Input: part model. Units: mm. Frame: model coordinates. Face numbers are marked on the shaded views. A direction names the side the tool comes from. Round coordinates to 2 decimals unless told otherwise and drop trailing zeros. Write each loop counter-clockwise with the first axis right and the second up, starting at its lowest first coordinate (ties: lowest second). Pieces come first, ordered by that corner, then holes. Notation, with made-up numbers: M -31,77 L 21,77 A33 ccw 21,105 Z; hole C -22,86.25 d10. An arc over 180 degrees is marked long. Use one line per item in the form item = value. Start each with the question number.
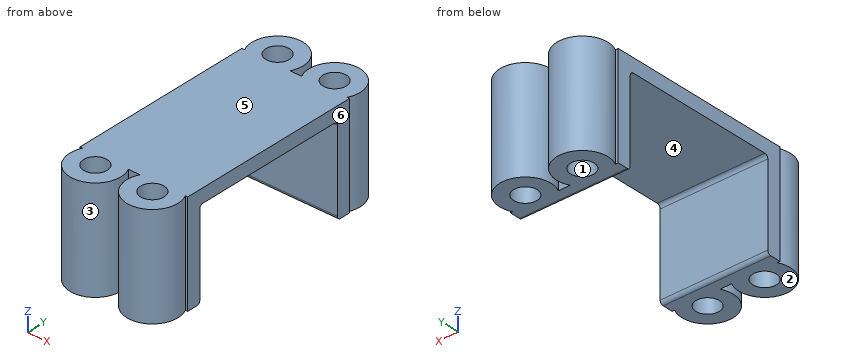
```python
from build123d import *

# Parameters (mm, degrees)
SCHIZZO1_W                   = 15.6
SCHIZZO1_H                   = 22.8
ESTRUSIONE_ESTRUSIONE1_DEPTH = 2
SCHIZZO7_R                   = 1.7
ESTRUSIONE_ESTRUSIONE8_DEPTH = 14.75
RACCORDO2_R                  = 0.5


with BuildPart() as part:
    # Schizzo1 → Estrusione-Estrusione1 (new body)
    with BuildSketch(Plane.XY):
        with Locations((-0.031567178, 0)):
            Rectangle(SCHIZZO1_W, SCHIZZO1_H)
    extrude(amount=ESTRUSIONE_ESTRUSIONE1_DEPTH)

    # Schizzo7 → Estrusione-Estrusione8 (add)
    # profile 1 of 2: a face of its own
    with BuildSketch(Plane.XY.offset(2)):
        with BuildLine():
            Line((7.768432822, 13.4), (7.417902523, 13.4))
            ThreePointArc((7.417902523, 13.4), (4.131567178, 18.8), (0.845231833, 13.4))
            Line((0.845231833, 13.4), (-0.845231833, 13.4))
            ThreePointArc((-0.845231833, 13.4), (-4.131567178, 18.8), (-7.417902523, 13.4))
            Line((-7.417902523, 13.4), (-7.831567178, 13.4))
            Line((-7.831567178, 13.4), (-7.831567178, 11.4))
            Line((-7.831567178, 11.4), (7.768432822, 11.4))
            Line((7.768432822, 11.4), (7.768432822, 13.4))
        make_face()
        with Locations((4.131567178, 15.1)):
            Circle(SCHIZZO7_R, mode=Mode.SUBTRACT)
        with Locations(Location((-4.131567178, 15.1, 0), (0, 0, 180))):
            Circle(SCHIZZO7_R, mode=Mode.SUBTRACT)
    # profile 2 of 2: a face of its own
    with BuildSketch(Plane.XY.offset(2)):
        with BuildLine():
            Line((0.845231833, -13.4), (-0.845231833, -13.4))
            ThreePointArc((-0.845231833, -13.4), (-4.131567178, -18.8), (-7.417902523, -13.4))
            Line((-7.417902523, -13.4), (-7.831567178, -13.4))
            Line((-7.831567178, -13.4), (-7.831567178, -11.4))
            Line((-7.831567178, -11.4), (7.768432822, -11.4))
            Line((7.768432822, -11.4), (7.768432822, -13.4))
            Line((7.768432822, -13.4), (7.417902523, -13.4))
            ThreePointArc((7.417902523, -13.4), (4.131567178, -18.8), (0.845231833, -13.4))
        make_face()
        with Locations((-4.131567178, -15.1)):
            Circle(SCHIZZO7_R, mode=Mode.SUBTRACT)
        with Locations(Location((4.131567178, -15.1, 0), (0, 0, 180))):
            Circle(SCHIZZO7_R, mode=Mode.SUBTRACT)
    extrude(amount=-ESTRUSIONE_ESTRUSIONE8_DEPTH)

    # Raccordo2
    raccordo2_edges = [part.edges().sort_by_distance(p)[0] for p in [
        (-0.031567178, 11.4, 0),
        (-0.031567178, 11.4, -12.75),
        (-0.031567178, -11.4, 0),
        (-0.031567178, -11.4, -12.75),
    ]]
    fillet(raccordo2_edges, radius=RACCORDO2_R)


solid = part.part
```
Item 1: Cut plane A-A (z = -1.75). Output: boundary loops of the cut face in (x, y), plus the area to 3 significant figures.
Item 2: Cut plane B-B (y = -15.1). Output: boundary loops of the cut face in (x, z).
Item 3: First-contact query: pin 1 (0.8 mm diameter, centred on x = 0, z = -5.5, fed in from -Y); pin 2 (8 mm diameter, centred on x = -4, y = 5, fed in from -Z); pin 3 (0.8 mm diameter, centred on x = 0, z = -5, fed in from +Y). Flat tips, straight axial feed; report the tip coordinate or a pass-through.
Item 4: Reachability of the marked faces 4, 5 and 6 from +Z, -Z, +X, -X, +Y, -Y: full face, straight path, thin tool, end or side. Return the list, or none.
Item 5: Cut plane C-C (x = -3.5). Output: boundary loops of the cut face in (y, z), plus the area to 3 significant figures.
Item 6: Ray query, line 1 (Y direction, x = 3.75, z = -1.25); line 2 (Z direction, x = 0.25, y = -9); line 3 (Y direction, x = -0.25, z = -10.25). Return the intervals inside material, ascending. Write a range as from..to.
Item 7: Draft query along Y for the marked faces 1, 2 and 3. Return one class per face: +Y half, -Y half, draft (parallel to the pull), parting line (faces both ways), or undercut.
Item 8: Cut plane D-D (x = 6.5). Output: boundary loops of the cut face in (y, z).
Final values:
q1.outline = M -7.83,-13.4 L -7.42,-13.4 A3.7 ccw long -0.85,-13.4 L 0.85,-13.4 A3.7 ccw long 7.42,-13.4 L 7.77,-13.4 L 7.77,-11.4 L -7.83,-11.4 Z; M -7.83,11.4 L 7.77,11.4 L 7.77,13.4 L 7.42,13.4 A3.7 ccw long 0.85,13.4 L -0.85,13.4 A3.7 ccw long -7.42,13.4 L -7.83,13.4 Z; hole C -4.13,-15.1 d3.4; hole C -4.13,15.1 d3.4; hole C 4.13,-15.1 d3.4; hole C 4.13,15.1 d3.4
q1.area = 161 mm^2
q2.outline = M -7.83,-12.75 L -5.83,-12.75 L -5.83,2 L -7.83,2 Z; M -2.43,-12.75 L -0.43,-12.75 L -0.43,2 L -2.43,2 Z; M 0.43,-12.75 L 2.43,-12.75 L 2.43,2 L 0.43,2 Z; M 5.83,-12.75 L 7.83,-12.75 L 7.83,2 L 5.83,2 Z
q3.pin_1 = -13.4
q3.pin_2 = 0
q3.pin_3 = 13.4
q4.face_4 = -Z, +X, -X
q4.face_5 = +Z, +X, -X, +Y, -Y
q4.face_6 = +Z, -Z, +X
q5.outline = M -18.75,-12.75 L -16.68,-12.75 L -16.68,2 L -18.75,2 Z; M -13.52,-12.75 L -11.9,-12.75 A0.5 ccw -11.4,-12.25 L -11.4,-0.5 A0.5 cw -10.9,0 L 10.9,0 A0.5 cw 11.4,-0.5 L 11.4,-12.25 A0.5 ccw 11.9,-12.75 L 13.52,-12.75 L 13.52,2 L -13.52,2 Z; M 16.68,-12.75 L 18.75,-12.75 L 18.75,2 L 16.68,2 Z
q5.area = 169 mm^2
q6.line_1 = -18.78..-16.76, -13.44..-11.4, 11.4..13.44, 16.76..18.78
q6.line_2 = 0..2
q6.line_3 = -13.4..-11.4, 11.4..13.4
q7.face_1 = undercut
q7.face_2 = draft
q7.face_3 = undercut
q8.outline = M -17.94,-12.75 L -11.9,-12.75 A0.5 ccw -11.4,-12.25 L -11.4,-0.5 A0.5 cw -10.9,0 L 10.9,0 A0.5 cw 11.4,-0.5 L 11.4,-12.25 A0.5 ccw 11.9,-12.75 L 17.94,-12.75 L 17.94,2 L -17.94,2 Z
